The model under review builds one solid part; all positions refer to its coordinate system, in mm. Face numbers are marked on the shaded views. A direction names the side the tool comes from. Coordinates: 2 decimals unless noted, no trailing zeros. Loops run counter-clockwise (first coordinate to the right, second up) from the corner with the lowest first, then second, coordinate; pieces in that order, holes last. Notation, with made-up numbers: (34, 15) -> (56, 15) arc R26 cw to (56, 38) -> close; hole circle Ø7 at (-4, -33.5). An arc over 180 degrees is marked (long way). One line per question, with ' | ' between items. Start each with the question number.
from build123d import *

# Parameters (mm, degrees)
SKETCH006_R             = 2.5
PAD005_DEPTH            = 8
PAD006_DEPTH            = 5
FILLET_R                = 4
FILLET001_R             = 1
BODY001_PLACEMENT_ANGLE = 90


with BuildPart() as part:
    # Sketch006 → Pad005 (new body)
    with BuildSketch(Plane.XZ):
        with BuildLine():
            ThreePointArc((0, 7), (-4.1833, -5.612486), (6.708204, 2))
            Line((60, 2), (6.708204, 2))
            Line((60, 7), (60, 2))
            Line((0, 7), (60, 7))
        make_face()
        Circle(SKETCH006_R, mode=Mode.SUBTRACT)
    extrude(amount=PAD005_DEPTH)

    # Sketch007 (on Face4 of Pad005) → Pad006 (join)
    with BuildSketch(Plane.XY.offset(2)):
        Polygon((20, 0), (25, 8), (60, 8), (60, -16), (25, -16), (20, -8), align=None)
    extrude(amount=PAD006_DEPTH)

    # Fillet
    fillet_edges = [part.edges().sort_by_distance(p)[0] for p in [
        (25, 8, 4.5),
        (25, -16, 4.5),
        (20, -8, 4.5),
        (20, 0, 4.5),
    ]]
    fillet(fillet_edges, radius=FILLET_R)

    # Fillet001
    fillet001_edges = [part.edges().sort_by_distance(p)[0] for p in [
        (60, 8, 4.5),
        (60, -16, 4.5),
    ]]
    fillet(fillet001_edges, radius=FILLET001_R)


with BuildPart() as part_1:
    # Body001 placement: moved
    add(part.part.moved(Location((-4, -10.5, 11.5))).rotate(Axis((-4, -10.5, 11.5), (0, 0, 1)), BODY001_PLACEMENT_ANGLE))


solid = part_1.part
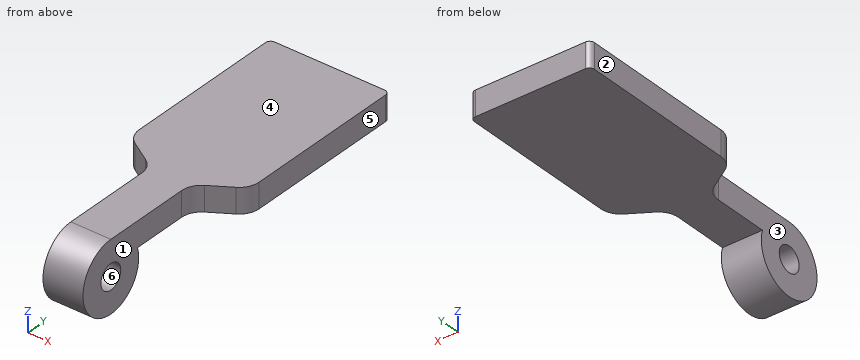
1) Machinability: for the marked faces 1, 2 and 3, which of the approach directions +Z, -Z, +X, -X, +Y, -Y give a long, thin tool a straight path to every point of the face, cutting with its end or side? Answer none if there is none.
2) Insertion check: pin 1 Ø1.5 at (x, y) = (-8, 13.5) entering from -Z; pin 2 Ø8 at (y, z) = (-2, 14) entering from +X; pin 3 Ø6.5 at (y, z) = (-10.5, 11.5) entering from -X. Each pin has a flat end and moves straight along its axis. Give the tip position at first contact, or say it passes through.
3) Consider section A-A, the plane z = 11.5. Write out the cut boundary in (x, y), plus the area to 3 significant figures.
4) Consider section B-B, the plane x = -0.5. Write out the cut boundary in (y, z), plus the area to 3 significant figures.
5) Consider section D-D, the plane y = 29.5. Write out the cut boundary in (x, z).
6) Consider section C-C, the plane z = 16.75. Write out the cut boundary in (x, y) (3 decimals).
7) Wall thickness on L1, parallel to Z at x = 0.5, y = -10.5; L2, parallel to Z at x = -3.25, y = 32; L3, parallel to X at y = -2.5, z = 13.75: over which ranges is each line inside the solid? List them lowest first.
8) Mouldability with a two-part tool opening along Z and no side actions: class the marked faces 4, 5 and 6 as +Z half, -Z half, draft (parallel to the pull), parting line (faces both ways), or undercut.
Filled sheet:
1) face 1: +Z, -Z, +X, -Y | face 2: +Z, -Z, -X, +Y, -Y | face 3: +Z, -Z, -X, -Y
2) pin 1: z = 13.5 | pin 2: x = 4 | pin 3: x = -4
3) outline: (-4, -17.5) -> (4, -17.5) -> (4, -13) -> (-4, -13) -> close; (-4, -8) -> (4, -8) -> (4, -3.5) -> (-4, -3.5) -> close | area: 72.0 mm^2
4) outline: (-10.5, 18.5) arc R7 ccw (long way) to (-3.79, 13.5) -> (49.5, 13.5) -> (49.5, 18.5) -> close; hole circle Ø5 at (-10.5, 11.5) | area: 410 mm^2
5) outline: (-12, 13.5) -> (12, 13.5) -> (12, 18.5) -> (-12, 18.5) -> close
6) outline: (-12, 16.717) arc R4 ccw to (-10.12, 13.325) -> (-5.88, 10.675) arc R4 cw to (-4, 7.283) -> (-4, -15.13) -> (4, -15.13) -> (4, 7.283) arc R4 cw to (5.88, 10.675) -> (10.12, 13.325) arc R4 ccw to (12, 16.717) -> (12, 48.5) arc R1 ccw to (11, 49.5) -> (-11, 49.5) arc R1 ccw to (-12, 48.5) -> close
7) L1: 4.5 to 9, 14 to 18.5 | L2: 13.5 to 18.5 | L3: -4 to 4
8) face 4: +Z half | face 5: draft | face 6: undercut
